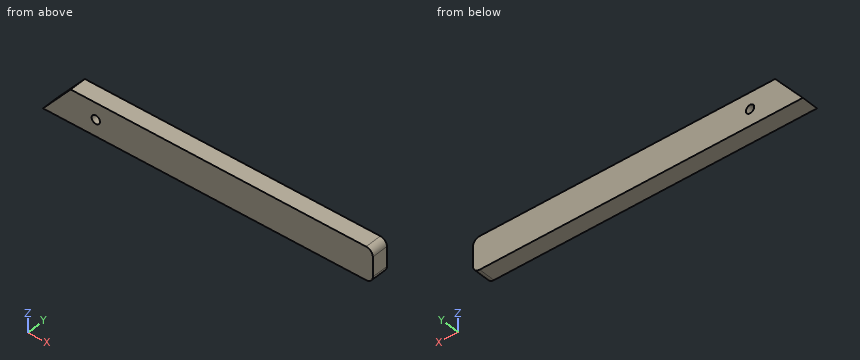
```python
from build123d import *

# Parameters (mm, degrees)
F0_R     = 3.175
F1_DEPTH = 12.7
F2_R     = 5.08
F3_R     = 5.08


with BuildPart() as f1:
    # F0 (on Front) → F1 (new body)
    with BuildSketch(Plane.XZ):
        Polygon((20.977491, 25), (0, 0), (250, 0), (250, 25), align=None)
        with Locations((40, 12.5)):
            Circle(F0_R, mode=Mode.SUBTRACT)
    extrude(amount=F1_DEPTH)

    # F2
    f2_edges = [f1.edges().sort_by_distance(p)[0] for p in [
        (250, -6.35, 25),
    ]]
    fillet(f2_edges, radius=F2_R)

    # F3
    f3_edges = [f1.edges().sort_by_distance(p)[0] for p in [
        (250, -6.35, 0),
    ]]
    fillet(f3_edges, radius=F3_R)


solid = f1.part
```
The listing builds one solid part. Answer for the finished solid, in the listing's coordinates (mm). Coordinates: 2 decimals unless noted, no trailing zeros. Write each loop counter-clockwise with the first axis right and the second up, starting at its lowest first coordinate (ties: lowest second). Pieces come first, ordered by that corner, then holes. Notation, with made-up numbers: (3, 23) -> (52, 23) arc R23 ccw to (52, 58) -> close; hole circle Ø5 at (-11.5, 30). An arc over 180 degrees is marked (long way). Write each question's results on one line, items separated by ' | '. Start each with the question number.
1) Straight lines are drawn through the part: probe 1 along Z at (x, y) = (40, -8.5) (3 decimals); probe 2 along X at (y, z) = (-8, 14); probe 3 along X at (y, z) = (-0.5, 6). For each, find the intervals that lie inside material, in ascending order.
2) A cutting plane is placed at A-A (x = 40). Determine the outline of the cut face in (y, z) (3 decimals).
3) Flat-ended cylindrical pins translate along their axes: pin 1 Ø2 at (y, z) = (-7, 4) entering from -X; pin 2 Ø5.5 at (x, z) = (40, 12.5) entering from -Y. Find the tip coordinate at first contact, or state that the pin passes through.
4) A cutting plane is placed at C-C (z = 12.5). Determine the outline of the cut face in (x, y) (3 decimals), then the cut area to 3 significant figures.
5) A cutting plane is placed at D-D (z = 22.75). Determine the outline of the cut face in (x, y), then the cut area to 3 significant figures.
Values follow:
1) probe 1: 0 to 9.325, 15.675 to 25 | probe 2: 11.75 to 37.2, 42.8 to 250 | probe 3: 5.03 to 250
2) outline: (-12.7, 0) -> (0, 0) -> (0, 9.325) -> (-12.7, 9.325) -> close; (-12.7, 15.675) -> (0, 15.675) -> (0, 25) -> (-12.7, 25) -> close
3) pin 1: x = 2.52 | pin 2: through
4) outline: (10.489, -12.7) -> (36.825, -12.7) -> (36.825, 0) -> (10.489, 0) -> close; (43.175, -12.7) -> (250, -12.7) -> (250, 0) -> (43.175, 0) -> close | area: 2,960 mm²
5) outline: (19.09, -12.7) -> (249.14, -12.7) -> (249.14, 0) -> (19.09, 0) -> close | area: 2,920 mm²
